Drawing for the job (mm, zero at the part's lowest x, y, z). Coordinates: 2 decimals unless noted, no trailing zeros. Order: outer loops, then holes, each group sorted by start corner. A loop starts at its lowest first (then second) coordinate and runs counter-clockwise, first axis right, second up.
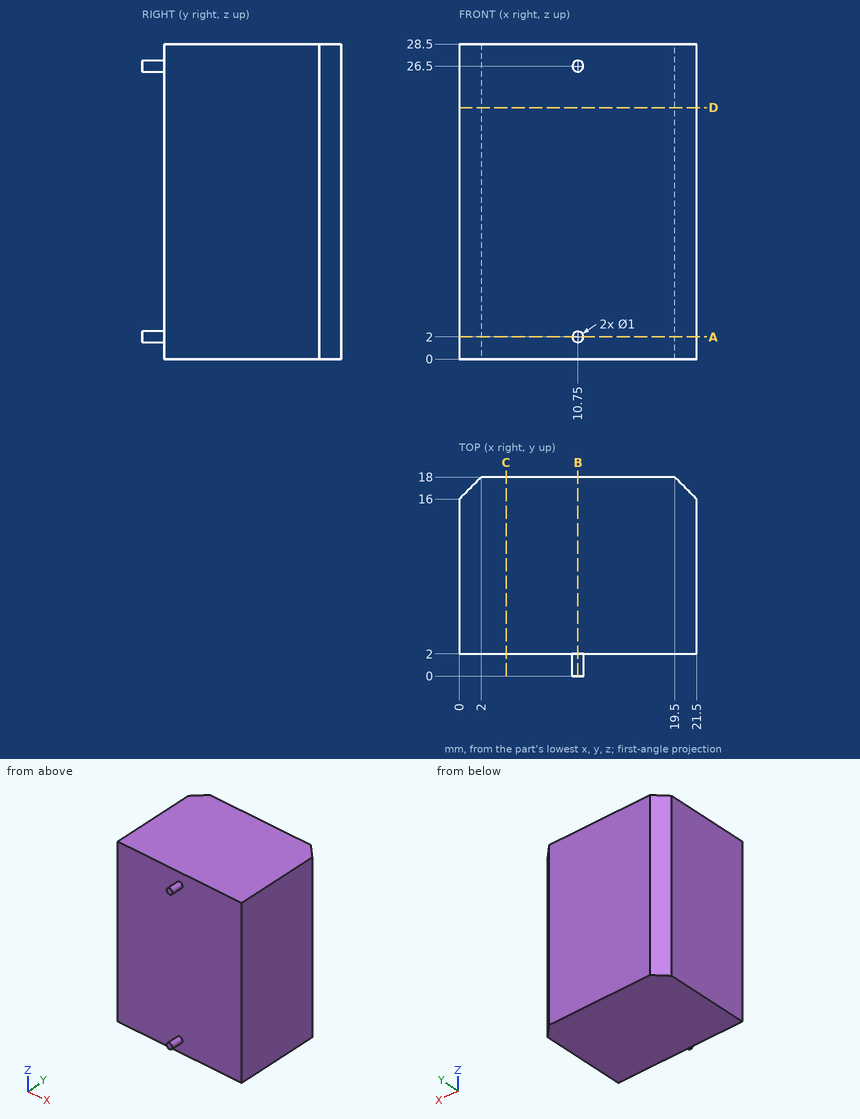
(1) Slice it at D-D, the plane z = 22.75. Give the cut face in (x, y), then the cut area to 3 significant figures.
(2) Drop a flat-ended pin along its axis: pin 1 (1.5 mm diameter, centred on x = 10, z = 16, fed in from -Y). Give the stop position or say it passes through.
(3) Slice it at A-A, the plane z = 2. Give the cut face in (x, y), then the cut area to 3 significant figures.
(4) Slice it at B-B, the plane x = 10.75. Give the cut face in (y, z).
(5) Probe line 1 (Y direction, x = 18.25, z = 2.5); line 2 (X direction, y = 16.25, z = 22.75); line 3 (X direction, y = 16.5, z = 26.75). List the from-to ranges inside material, lowest first.
(6) Slice it at C-C, the plane x = 4.25. Give the cut face in (y, z).
Here are the results:
1. outline: (0, 2) - (21.5, 2) - (21.5, 16) - (19.5, 18) - (2, 18) - (0, 16) - close
1. area: 340 mm2
2. pin 1: stops at y = 2
3. outline: (0, 2) - (10.25, 2) - (10.25, 0) - (11.25, 0) - (11.25, 2) - (21.5, 2) - (21.5, 16) - (19.5, 18) - (2, 18) - (0, 16) - close
3. area: 342 mm2
4. outline: (0, 1.5) - (2, 1.5) - (2, 0) - (18, 0) - (18, 28.5) - (2, 28.5) - (2, 27) - (0, 27) - (0, 26) - (2, 26) - (2, 2.5) - (0, 2.5) - close
5. line 1: y = 2 to 18
5. line 2: x = 0.25 to 21.25
5. line 3: x = 0.5 to 21
6. outline: (2, 0) - (18, 0) - (18, 28.5) - (2, 28.5) - close
